Build history of the part. All positions in model axes, mm. A direction names the side the tool comes from. Give positions to 0.01 mm unless a question says otherwise; leave off trailing zeros. Write each loop counter-clockwise with the first axis right and the second up, starting at its lowest first coordinate (ties: lowest second). Pieces come first, ordered by that corner, then holes. Notation, with made-up numbers: M 29.25,68 L 73.25,68 A5 cw 73.25,76 Z; hole C -10,-22 d8. An arc over 180 degrees is marked long. Return JSON: item names as keys, results as strings. Group by question number.
Q1. Wall check: probe 1 along Z at (x, y) = (9.5, -1.15); probe 2 along Y at (x, z) = (9, -2.5); probe 3 along Y at (x, z) = (2.5, -6.75). Give the ranges that are in metal, low to high.
Q2. Band-saw the part on D-D, the plane z = -5.75. Give the cut face in (x, y).
Q3. Band-saw the part on A-A, the plane x = 11.75. Give the cut face in (y, z), then the cut area to 3 significant figures.
Q4. Flat gauge pins, fed straight in: pin 1 Ø2 at (x, y) = (10.5, -0.5) entering from +Z; pin 2 Ø1.5 at (x, z) = (8.5, -1) entering from -Y; pin 3 Ø1.8 at (x, z) = (9.5, -4) entering from -Y. Where does each tip first touch, or does it go through?
Q5. Tool access for faces 1 (the flat face through (10, -1, -6.9)), 2 (the flat face through (10, 3, -4)): list every direction of +Z, -Z, +X, -X, +Y, -Y with a clear straight run to the whole face (end or side of a thin tool).
Q6. Band-saw the part on C-C, the plane x = 6. Give the cut face in (y, z).
Q7. Band-saw the part on B-B, the plane z = -4. Give the cut face in (x, y).
Q8. Pull direction Z, two halves, no side cores. Call faces 3 (the flat face through (10, 0, -6)), 4 (the cylindrical face through (9.561, 0.394, -5.413)), 5 (the flat face through (10, 0.8, -4)), 6 (the flat face through (10.1, 1.5, -7.7)): +Z half, -Z half, draft (parallel to the pull), parting line (faces both ways), or undercut.
from build123d import *

# Parameters (mm, degrees)
SKETCH1_W               = 20.5
SKETCH1_H               = 8
BOSS_EXTRUDE1_DEPTH     = 3
CUT_EXTRUDE1_DEPTH      = 23.209232315
CUT_EXTRUDE1_DEPTH_BACK = 23.209232315
CUT_EXTRUDE2_DEPTH      = 23.209232315
CUT_EXTRUDE2_DEPTH_BACK = 23.209232315
SKETCH4_R               = 1.8
CUT_EXTRUDE3_DEPTH      = 0.8
SKETCH5_W               = 8
SKETCH5_H               = 1.1
BOSS_EXTRUDE2_DEPTH     = 2
FILLET1_R               = 4


with BuildPart() as part:
    # Sketch1 → Boss-Extrude1 (new body)
    with BuildSketch(Plane(origin=(0, 0, 0), x_dir=(1, 0, 0), z_dir=(0, 1, 0))):
        with Locations((10.25, 4)):
            Rectangle(SKETCH1_W, SKETCH1_H)
    extrude(amount=BOSS_EXTRUDE1_DEPTH)

    # Sketch2 → Cut-Extrude1 (cut, two sides: drawn at the far end of the back side and taken through both)
    with BuildSketch(Plane.XY.offset(-CUT_EXTRUDE1_DEPTH_BACK)):
        Polygon((0, 0), (0.6, 3), (0, 3), align=None)
        Polygon((20.5, 0), (19.9, 3), (20.5, 3), align=None)
    extrude(amount=CUT_EXTRUDE1_DEPTH + CUT_EXTRUDE1_DEPTH_BACK, mode=Mode.SUBTRACT)

    # Sketch3 → Cut-Extrude2 (cut, two sides: drawn at the far end of the back side and taken through both)
    with BuildSketch(Plane(origin=(0, 0, 0), x_dir=(0, 0, -1), z_dir=(1, 0, 0)).offset(-CUT_EXTRUDE2_DEPTH_BACK)):
        Polygon((0, 0), (0.6, 3), (0, 3), align=None)
        Polygon((8, 3), (7.4, 3), (8, 0), align=None)
    extrude(amount=CUT_EXTRUDE2_DEPTH + CUT_EXTRUDE2_DEPTH_BACK, mode=Mode.SUBTRACT)

    # Sketch4 → Cut-Extrude3 (cut)
    with BuildSketch(Plane.XZ):
        with Locations(Location((10.25000125, -3.75, 0), (0, 0, 270))):
            Circle(SKETCH4_R)
    extrude(amount=-CUT_EXTRUDE3_DEPTH, mode=Mode.SUBTRACT)

    # Sketch5 → Boss-Extrude2 (add)
    with BuildSketch(Plane.XZ):
        with Locations((10.250011, -7.45)):
            Rectangle(SKETCH5_W, SKETCH5_H)
    extrude(amount=BOSS_EXTRUDE2_DEPTH)

    # Fillet1
    # the kernel refuses this fillet: 4 mm, written as the material it takes off along each edge
    with BuildSketch(Plane(origin=(14.250011, -2, -16.660254038), x_dir=(0, 1, 0), z_dir=(0, 0, 1)), Plane(origin=(6.250011, -2, 1.760254038), x_dir=(0, 1, 0), z_dir=(0, 0, -1))) as fillet1_piece_1:
        with BuildLine():
            CenterArc((4, 3.464101615), FILLET1_R, 180, 60)
            Line((0, 3.464101615), (-0.08, 3.464101615))
            Line((-0.08, 3.464101615), (-0.08, 0))
            Line((-0.08, 0), (0, -0.08))
            ThreePointArc((0, -0.08), (1, -0.08), (1.96, -0.069282032))
            Line((1.96, -0.069282032), (2, 0))
        make_face()
    extrude(amount=18.420508076, mode=Mode.SUBTRACT)


solid = part.part
From the geometry:
{
 "1": {"probe 1": "z = -8 to -6.9", "probe 2": "y = 0.8 to 3", "probe 3": "y = 0 to 3"},
 "2": {"outline": "M 0,0 L 20.5,0 L 19.9,3 L 0.6,3 Z"},
 "3": {"outline": "M -1.88,-8 L 0,-8 L 3,-7.4 L 3,-0.6 L 0,0 L 0,-2.76 L 0.8,-2.76 L 0.8,-4.74 L 0,-4.74 L 0,-6.9 L -1.88,-6.9 Z", "area": "22.7 mm^2"},
 "4": {"pin 1": "stops at z = 0", "pin 2": "stops at y = 0", "pin 3": "stops at y = 0.8"},
 "5": {"face 1": "+Z, +X, -X, -Y", "face 2": "+Z, -Z, +X, -X, +Y"},
 "6": {"outline": "M 0,-8 L 3,-7.4 L 3,-0.6 L 0,0 Z"},
 "7": {"outline": "M 0,0 L 8.47,0 L 8.47,0.8 L 12.03,0.8 L 12.03,0 L 20.5,0 L 19.9,3 L 0.6,3 Z"},
 "8": {"face 3": "draft", "face 4": "undercut", "face 5": "undercut", "face 6": "-Z half"}
}
